```python
from build123d import *
from build123d.topology import SkipClean

# Parameters (mm, degrees)
BOSS_EXTRUDE1_DEPTH = 2
SKETCH2_R           = 3.5
SKETCH2_R_2         = 2.25
BOSS_EXTRUDE2_DEPTH = 3.5
SKETCH3_R           = 1.25
CUT_EXTRUDE1_DEPTH  = 5
SKETCH4_R           = 2.5
CUT_EXTRUDE2_DEPTH  = 1
SKETCH5_R           = 0.5
CUT_EXTRUDE3_DEPTH  = 5


with BuildPart() as part:
    # Sketch1 → Boss-Extrude1 (new body)
    with BuildSketch(Plane(origin=(0, 0, 0), x_dir=(1, 0, 0), z_dir=(0, 1, 0))):
        with BuildLine():
            Line((-14.25, 1.75), (-2.449489743, 2.5))
            ThreePointArc((-2.449489743, 2.5), (0, 3.5), (2.449489743, 2.5))
            Line((2.449489743, 2.5), (14.25, 1.75))
            ThreePointArc((14.25, 1.75), (16, 0), (14.25, -1.75))
            Line((14.25, -1.75), (2.449489743, -2.5))
            ThreePointArc((2.449489743, -2.5), (0, -3.5), (-2.449489743, -2.5))
            Line((-2.449489743, -2.5), (-14.25, -1.75))
            ThreePointArc((-14.25, -1.75), (-16, 0), (-14.25, 1.75))
        make_face()
    extrude(amount=BOSS_EXTRUDE1_DEPTH)

    # Sketch2 → Boss-Extrude2 (add)
    with SkipClean():  # the faces are left unmerged after this step: merging them gives an invalid solid
        with BuildSketch(Plane(origin=(0, 2, 0), x_dir=(1, 0, 0), z_dir=(0, 1, 0))):
            with Locations(Location((0, 0, 0), (0, 0, 45.584691403))):
                Circle(SKETCH2_R)
            with Locations(Location((0, 0, 0), (0, 0, 270))):
                Circle(SKETCH2_R_2, mode=Mode.SUBTRACT)
        extrude(amount=BOSS_EXTRUDE2_DEPTH)

    # Sketch3 → Cut-Extrude1 (cut)
    with SkipClean():  # the faces are left unmerged after this step: merging them gives an invalid solid
        with BuildSketch(Plane(origin=(0, 2, 0), x_dir=(1, 0, 0), z_dir=(0, 1, 0))):
            with Locations(Location((0, 0, 0), (0, 0, 270))):
                Circle(SKETCH3_R)
        extrude(amount=-CUT_EXTRUDE1_DEPTH, mode=Mode.SUBTRACT)

    # Sketch4 → Cut-Extrude2 (cut)
    with SkipClean():  # the faces are left unmerged after this step: merging them gives an invalid solid
        with BuildSketch(Plane.XZ):
            with Locations(Location((0, 0, 0), (0, 0, 270))):
                Circle(SKETCH4_R)
        extrude(amount=-CUT_EXTRUDE2_DEPTH, mode=Mode.SUBTRACT)

    # Sketch5 → Cut-Extrude3 (cut)
    with SkipClean():  # the faces are left unmerged after this step: merging them gives an invalid solid
        with BuildSketch(Plane.XZ):
            with Locations(Location((14.25, 0, 0), (0, 0, 270))):
                Circle(SKETCH5_R)
            with Locations(Location((12.25, 0, 0), (0, 0, 270))):
                Circle(SKETCH5_R)
            with Locations(Location((10.25, 0, 0), (0, 0, 270))):
                Circle(SKETCH5_R)
            with Locations(Location((8.25, 0, 0), (0, 0, 270))):
                Circle(SKETCH5_R)
            with Locations(Location((6.25, 0, 0), (0, 0, 270))):
                Circle(SKETCH5_R)
            with Locations(Location((4.25, 0, 0), (0, 0, 270))):
                Circle(SKETCH5_R)
            with Locations(Location((-14.25, 0, 0), (0, 0, 270))):
                Circle(SKETCH5_R)
            with Locations(Location((-12.25, 0, 0), (0, 0, 90))):
                Circle(SKETCH5_R)
            with Locations(Location((-10.25, 0, 0), (0, 0, 90))):
                Circle(SKETCH5_R)
            with Locations(Location((-8.25, 0, 0), (0, 0, 90))):
                Circle(SKETCH5_R)
            with Locations(Location((-6.25, 0, 0), (0, 0, 90))):
                Circle(SKETCH5_R)
            with Locations(Location((-4.25, 0, 0), (0, 0, 90))):
                Circle(SKETCH5_R)
        extrude(amount=-CUT_EXTRUDE3_DEPTH, mode=Mode.SUBTRACT)


solid = part.part
```
Build history of the part. All positions in model axes, mm. A direction names the side the tool comes from. Round coordinates to 2 decimals unless told otherwise and drop trailing zeros. Order: outer loops, then holes, each group sorted by start corner. A loop starts at its lowest first (then second) coordinate and runs counter-clockwise, first axis right, second up. Notation, with made-up numbers: (85.25, -17.75) - (108.25, -17.75) arc R17 ccw to (108.25, 6.25) - close; hole circle Ø3 at (49, -14.75). An arc over 180 degrees is marked (long way). Use a Markdown table: item, result.
1) Flat gauge pins, fed straight in: pin 1 Ø1 at (x, z) = (9.5, 0.5) entering from -Y; pin 2 Ø3 at (x, y) = (-7, 2) entering from -Z; pin 3 Ø4 at (x, z) = (0, 0) entering from +Y; pin 4 Ø1.5 at (x, z) = (-1, 0) entering from -Y. Where does each tip first touch, or does it go through?
Recorded:
| item | result |
|---|---|
| pin 1 | stops at y = 0 |
| pin 2 | stops at z = -2.31 |
| pin 3 | stops at y = 2 |
| pin 4 | stops at y = 1 |
2) Saw through at C-C on y = 4.25. Write the cut outline in (x, z), and give its area (3 significant figures).
Recorded:
| item | result |
|---|---|
| outline | circle Ø7 at (0, 0); hole circle Ø4.5 at (0, 0) |
| area | 22.6 mm² |
3) Saw through at D-D on x = 4.25. Write the cut outline in (y, z).
Recorded:
| item | result |
|---|---|
| outline | (0, -2.39) - (2, -2.39) - (2, -0.5) - (0, -0.5) - close; (0, 0.5) - (2, 0.5) - (2, 2.39) - (0, 2.39) - close |
4) Saw through at B-B on x = -10.25. Write the cut outline in (y, z), and give its area (3 significant figures).
Recorded:
| item | result |
|---|---|
| outline | (0, -2) - (2, -2) - (2, -0.5) - (0, -0.5) - close; (0, 0.5) - (2, 0.5) - (2, 2) - (0, 2) - close |
| area | 6.02 mm² |
5) Pull direction X, two halves, no side cores. Call faces 1 (the face through (-4.746, 0.986, -0.065)), 2 (the face through (2, 5.5, 2)), 3 (the face through (-2.44, 0.49, 0.54)), 4 (the face through (-8.27, 0.99, 2.13)): pulls with the +X half, pulls with the -X half, needs draft (parallel to the pull), parting line crosses it, or undercut.
Recorded:
| item | result |
|---|---|
| face 1 | undercut |
| face 2 | needs draft |
| face 3 | undercut |
| face 4 | pulls with the -X half |
6) Tool access for faces 5 (the face through (-1, 2, 1)), 6 (the face through (16, 1, 0)): list every direction of +Z, -Z, +X, -X, +Y, -Y with a clear straight run to the whole face (end or side of a thin tool).
Recorded:
| item | result |
|---|---|
| face 5 | +Y |
| face 6 | +X, +Y, -Y |
7) Saw through at A-A on y = 1.6. Give the number of separate pieces and of enclosed holes in the cut face, and give its area (3 significant figures).
Recorded:
| item | result |
|---|---|
| separate pieces | 1 |
| enclosed holes | 13 |
| area | 127 mm² |
8) Wall check: L1, parallel to X at y = 3.25, z = 0; L2, parallel to Y at x = 4.5, z = 2; L3, parallel to X at y = 3.9, z = 1.25. Give the ranges that are in metal, low to high.
Recorded:
| item | result |
|---|---|
| L1 | x = -3.5 to -2.25, 2.25 to 3.5 |
| L2 | y = 0 to 2 |
| L3 | x = -3.27 to -1.87, 1.87 to 3.27 |
